For this review, take the finished solid that the model builds, in its own axes (mm). A direction names the side the tool comes from. Give positions to 0.01 mm unless a question says otherwise; leave off trailing zeros. Order: outer loops, then holes, each group sorted by start corner. A loop starts at its lowest first (then second) coordinate and runs counter-clockwise, first axis right, second up.
Item 1: Consider section B-B (x = 19). Give the boundary of the cut face in (y, z) (1 decimal), plus the area to 3 significant figures.
Item 2: For probe 1 along X at (y, z) = (6, -8.5) (3 decimals); probe 2 along X at (y, z) = (-5, 5) (3 decimals); probe 3 along Y at (x, z) = (-21, 6.75), list the stretches that pass through material, from the lowest coordinate up.
Item 3: Consider section C-C (y = -2.25). Give the boundary of the cut face in (x, z) (3 decimals).
Item 4: Machinability: for faces 1 (the flat face through (15.875, 8, 0)), 2 (the flat face through (-15.875, 8, 0)), 3 (the flat face through (0, -9.5, 0)), which of the approach directions +Z, -Z, +X, -X, +Y, -Y give a long, thin tool a straight path to every point of the face, cutting with its end or side? Answer none if there is none.
Item 5: Consider section A-A (z = -5.5). Give the boundary of the cut face in (x, y) (3 decimals), plus the area to 3 significant figures.
Item 6: For P1, Ø2, axis at y = 6.5, z = 2.5, coming from the -X side; P2, Ø4, axis at y = 6.5, z = -3.5, coming from the -X side; P3, Ø1.8, axis at y = 7.5, z = -4, coming from the +X side (3 decimals), all flat-tipped, find the tip position at first contact; note any pin that passes through.
```python
from build123d import *

# Parameters (mm, degrees)
SKETCH1_W           = 31.75
SKETCH1_H           = 19
BOSS_EXTRUDE1_DEPTH = 9.525
BOSS_EXTRUDE2_DEPTH = 19.05
FILLET5_R           = 1


with BuildPart() as part:
    # Sketch1 → Boss-Extrude1 (new body, symmetric)
    with BuildSketch(Plane.XY):
        Rectangle(SKETCH1_W, SKETCH1_H)
    extrude(amount=BOSS_EXTRUDE1_DEPTH, both=True)

    # Sketch3 → Boss-Extrude2 (add)
    with BuildSketch(Plane.XY.offset(9.525)):
        Polygon((-15.875, -9.5), (-25.875, -9.5), (-15.875, 5.5), align=None)
        Polygon((15.875, -9.5), (15.875, 5.5), (25.875, -9.5), align=None)
    extrude(amount=-BOSS_EXTRUDE2_DEPTH)

    # Fillet5
    fillet5_edges = [part.edges().sort_by_distance(p)[0] for p in [
        (-25.875, -9.5, 0),
        (-15.875, 5.5, 0),
        (15.875, 5.5, 0),
        (25.875, -9.5, 0),
    ]]
    fillet(fillet5_edges, radius=FILLET5_R)


solid = part.part
```
Resolved:
1. outline: (-9.5, -9.5) - (0.8, -9.5) - (0.8, 9.5) - (-9.5, 9.5) - close
1. area: 196 mm2
2. probe 1: x = -15.875 to 15.875
2. probe 2: x = -22.875 to 22.875
2. probe 3: y = -9.5 to -2.19
3. outline: (-21.042, -9.525) - (21.042, -9.525) - (21.042, 9.525) - (-21.042, 9.525) - close
4. face 1: +Z, -Z, +X, +Y
4. face 2: +Z, -Z, -X, +Y
4. face 3: +Z, -Z, +X, -X, -Y
5. outline: (-24.839, -7.945) arc R1 ccw to (-24.006, -9.5) - (24.006, -9.5) arc R1 ccw to (24.839, -7.945) - (16.043, 5.248) arc R1 cw to (15.875, 5.803) - (15.875, 9.5) - (-15.875, 9.5) - (-15.875, 5.803) arc R1 cw to (-16.043, 5.248) - close
5. area: 752 mm2
6. P1: stops at x = -15.92
6. P2: stops at x = -16.54
6. P3: stops at x = 15.875
